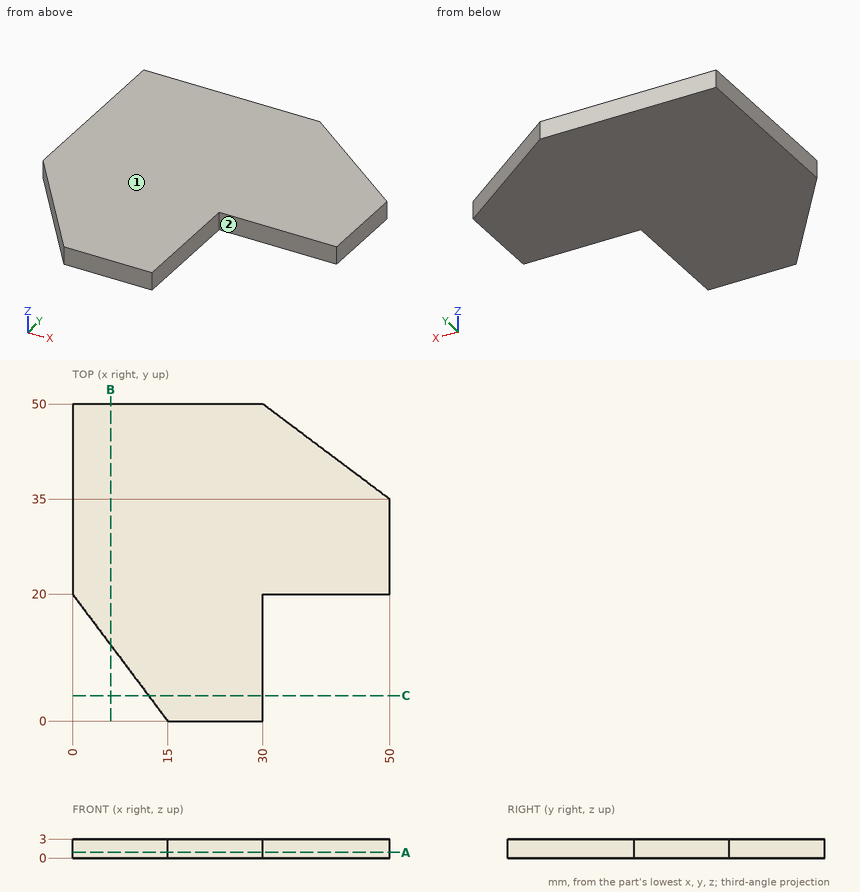
Could you check a few things on this drawing? It's one solid part, dimensions in mm from its lowest x, y, z. A direction names the side the tool comes from. Give positions to 0.01 mm unless a question says otherwise; leave off trailing zeros. Order: outer loops, then holes, each group sorted by start corner. A loop starts at its lowest first (then second) coordinate and runs counter-clockwise, first axis right, second up. Notation, with made-up numbers: (89.25, 60) - (105.25, 60) arc R20 cw to (105.25, 84) - close; hole circle Ø11 at (10, -28.5). An arc over 180 degrees is marked (long way). Answer as a JSON object with one key per item and string values. Group by question number.
Item 1: Which directions (+Z, -Z, +X, -X, +Y, -Y) give clear straight access to the entire face, cutting with the end or side of a thin tool? Please do the marked faces 1 and 2.
Item 2: If we section it at A-A on z = 0.9: Please give me the cut outline in (x, y).
Item 3: For P1, Ø1, axis at y = 13.5, z = 0.5, coming from the -X side; P2, Ø1.5, axis at x = 8, z = 2, coming from the -Y side; P3, Ø1.5, axis at x = 37, z = 1, coming from the -Y side, each with a flat end and sliding along its axis, tell me the tip position at first contact or that it passes through.
Item 4: If we section it at C-C on y = 4: Please give me the cut outline in (x, z), and give its area (3 significant figures).
Item 5: Please list where these lines run through material, in increasing order: probe 1 along X at (y, z) = (7, 2.95); probe 2 along X at (y, z) = (15, 1.45); probe 3 along Y at (x, z) = (6, 0.4).
Item 6: If we section it at B-B on x = 6: Please give me the cut outline in (y, z), and give its area (3 significant figures).
Result set:
{
 "1": {"face 1": "+Z, +X, -X, +Y, -Y", "face 2": "+Z, -Z, +X, -Y"},
 "2": {"outline": "(0, 20) - (15, 0) - (30, 0) - (30, 20) - (50, 20) - (50, 35) - (30, 50) - (0, 50) - close"},
 "3": {"P1": "x = 4.5", "P2": "y = 8.33", "P3": "y = 20"},
 "4": {"outline": "(12, 0) - (30, 0) - (30, 3) - (12, 3) - close", "area": "54.0 mm²"},
 "5": {"probe 1": "9.75 to 30", "probe 2": "3.75 to 30", "probe 3": "12 to 50"},
 "6": {"outline": "(12, 0) - (50, 0) - (50, 3) - (12, 3) - close", "area": "114 mm²"}
}
